Autodesk Inventor part; units mm, degrees
ref_plane "YZ Plane" through (0, 0, 0) normal (1, 0, 0) x (0, 1, 0)
ref_plane "XZ Plane" through (0, 0, 0) normal (0, 1, 0) x (-1, 0, 0)
ref_plane "XY Plane" through (0, 0, 0) normal (0, 0, 1) x (1, 0, 0)
sketch "Sketch1" plane through (0, 0, 0) normal (0, 0, 1) x (1, 0, 0)
  line L0 (0, 0) -> (0, 1910) construction
  line L1 (424.5155, 1910) -> (-415.4845, 1910)
  line L2 (-415.4845, 1910) -> (-1180, 1150)
  line L3 (-1180, 0) -> (-1180, 1150)
  line L4 (960, 0) -> (960, 1342.8524)
  line L5 (424.5155, 1910) -> (960, 1342.8524)
  circle A0 centre (0, 950) radius 195 construction
  line L6 (960, 0) -> (-1180, 0)
  circle A1 centre (-960, 220) radius 200
  circle A2 centre (-588, 255) radius 38
  circle A3 centre (374.6358, 1277) radius 50
  circle A4 centre (0, 950) radius 155
  point P0 (0, 955)
  dimension "d1" = 840
  dimension "d3" = 1150
  dimension "d11" = 390
  dimension "d12" = 1180
  dimension "d13" = 950
  dimension "d14" = 76
  dimension "d15" = 1910
  dimension "d16" = 255
  dimension "d17" = 220
  dimension "d18" = 400
  dimension "d19" = 220
  dimension "d21" = 1277
  dimension "d22" = 1554.6358
  dimension "d23" = 100
  dimension "d33" = 2140
  dimension "d34" = 494
  dimension "d45" = 310
  dimension "d49" = 372
  dimension "d51" = 780
  dimension "d52" = 1078
extrude "Extrusion1" add sketch "Sketch1" along normal blind 10
sketch "Sketch3" plane through (0, 0, 10) normal (0, 0, 1) x (1, 0, 0)
  line L0 (-400, 950) -> (400, 950) construction
  circle A0 centre (0, 950) radius 155
  circle A1 centre (155, 950) radius 2.5
  circle A2 centre (-155, 950) radius 2.5
  line L1 (132.7592, 870) -> (-132.7592, 870) construction
  circle A3 centre (132.7592, 870) radius 2.5
  circle A4 centre (-132.7592, 870) radius 2.5
  point P0 (0, 0)
  point P1 (-154.9798, 947.5001)
  point P2 (-154.9798, 952.4999)
  point P3 (154.9798, 947.5001)
  point P4 (154.9798, 952.4999)
  point P5 (134.0322, 872.1516)
  point P6 (131.4516, 867.8692)
  dimension "d47" = 5
  dimension "d48" = 80
extrude "Extrusion3" cut sketch "Sketch3" against normal through all contours A0 A1 | A0 A2 | A3 A0 | A4 A0 | A0 A4 picked at (155.7492, 949.3589) picked at (-155.8257, 950.101) picked at (133.5004, 869.6223)
sketch "Sketch4" plane through (0, 0, 10) normal (0, 0, 1) x (1, 0, 0)
  arc A0 (154.9798, 947.5001) -> (154.9798, 952.4999) centre (155, 950) ccw
  arc A1 (134.0322, 872.1516) -> (154.9798, 947.5001) centre (0, 950) ccw
  arc A2 (131.4516, 867.8692) -> (134.0322, 872.1516) centre (132.7592, 870) ccw
  arc A3 (-131.4516, 867.8692) -> (131.4516, 867.8692) centre (0, 950) ccw
  arc A4 (-134.0322, 872.1516) -> (-131.4516, 867.8692) centre (-132.7592, 870) ccw
  arc A5 (-154.9798, 947.5001) -> (-134.0322, 872.1516) centre (0, 950) ccw
  arc A6 (-154.9798, 952.4999) -> (-154.9798, 947.5001) centre (-155, 950) ccw
  arc A7 (154.9798, 952.4999) -> (-154.9798, 952.4999) centre (0, 950) ccw
  line L0 (960, 1342.8524) -> (424.5155, 1910)
  line L1 (424.5155, 1910) -> (-415.4845, 1910)
  line L2 (-415.4845, 1910) -> (-1180, 1150)
  line L3 (-1180, 1150) -> (-1180, 0)
  line L4 (-1180, 0) -> (960, 0)
  line L5 (960, 0) -> (960, 1342.8524)
  circle A8 centre (374.6358, 1277) radius 50
  circle A9 centre (-588, 255) radius 38
  circle A10 centre (-960, 220) radius 200
  line L6 (-380, 0) -> (-380, 1910)
  point P0 (0, 0)
  dimension "d53" = 1340
extrude "Extrusion4" cut sketch "Sketch4" against normal through all contours L6 L4 L3 L2 L1
equation "\"d17\" = d19"
properties part number "ДМФ 015 Стенка Нос ПРАВ"
The model under review builds one solid part; all positions refer to its coordinate system, in mm. A direction names the side the tool comes from. Round coordinates to 2 decimals unless told otherwise and drop trailing zeros. Loops run counter-clockwise (first coordinate to the right, second up) from the corner with the lowest first, then second, coordinate; pieces in that order, holes last. Notation, with made-up numbers: M 21,-32.75 L 68,-32.75 A34 ccw 68,6.25 Z; hole C 1,17.25 d4. An arc over 180 degrees is marked long. Write item = value, one per line.
Item 1: The part is to be moulded in two halves that separate along X. For faces 1 (the flat face through (281, 968, 10)), 2 (the cylindrical face through (397.708, 1321.359, 4.93)), 3 (the flat face through (688.509, 1630.396, 4.93)), say which applies: released by +X, released by -X, zero draft, split by the parting line, or undercut.
Return value:
face_1 = zero draft
face_2 = undercut
face_3 = released by +X
Item 2: Take a section at C-C on x = 0. Write out the cut boundary in (y, z), then the cut area to 3 significant figures.
Return value:
outline = M 0,0 L 795,0 L 795,10 L 0,10 Z; M 1105,0 L 1910,0 L 1910,10 L 1105,10 Z
area = 16,000 mm2
Item 3: Take a section at B-B on y = 1277. Write out the cut boundary in (x, z).
Return value:
outline = M -380,0 L 324.64,0 L 324.64,10 L -380,10 Z; M 424.64,0 L 960,0 L 960,10 L 424.64,10 Z
Item 4: Take a section at A-A on z = 4.75. Write out the cut boundary in (x, y).
Return value:
outline = M -380,0 L 960,0 L 960,1342.85 L 424.52,1910 L -380,1910 Z; hole M -154.98,947.5 A155 ccw -134.03,872.15 A2.5 ccw long -131.45,867.87 A155 ccw 131.45,867.87 A2.5 ccw long 134.03,872.15 A155 ccw 154.98,947.5 A2.5 ccw long 154.98,952.5 A155 ccw -154.98,952.5 A2.5 ccw long Z; hole C 374.64,1277 d100
Item 5: Machinability: for faces 4 (the flat face through (281, 968, 0)), 5 (the cylindrical face through (2.197, 795.016, 4.93)), which of the approach directions +Z, -Z, +X, -X, +Y, -Y give a long, thin tool a straight path to every point of the face, cutting with its end or side? Answer none if there is none.
Return value:
face_4 = -Z, +X, -X, +Y, -Y
face_5 = +Z, -Z
Item 6: For line 1 (X direction, y = 968.5, z = 6.75); line 2 (Y direction, x = 111.5, z = 0.5); line 3 (Y direction, x = 704, z = 6.25), list the stretches that pass through material, from the lowest coordinate up. Write a range as [from, to].
Return value:
line_1 = [-380, -153.89], [153.89, 960]
line_2 = [0, 842.33], [1057.67, 1910]
line_3 = [0, 1613.99]
Item 7: Take a section at D-D on y = 1488.5. Write out the cut boundary in (x, z), then the cut area to 3 significant figures.
Return value:
outline = M -380,0 L 822.48,0 L 822.48,10 L -380,10 Z
area = 12,000 mm2
Item 8: Insertion check: P1, Ø2, axis at y = 1589.5, z = 7.5, coming from the +X side. The pin has a flat end and moves straight along its axis. Give the tip position at first contact, or say it passes through.
Return value:
P1 = 728.07
